```python
from build123d import *

# Parameters (mm, degrees)
SKETCH1_R           = 24.1681
BOSS_EXTRUDE1_DEPTH = 69.7992
SKETCH2_R           = 20.2819
CUT_EXTRUDE1_DEPTH  = 78.718224606
SKETCH3_R           = 4.2164
CUT_EXTRUDE2_DEPTH  = 69.7992
SKETCH4_R           = 4.2164
CUT_EXTRUDE3_DEPTH  = 69.7992


with BuildPart() as part:
    # Sketch1 → Boss-Extrude1 (new body)
    with BuildSketch(Plane(origin=(0, 0, 0), x_dir=(1, 0, 0), z_dir=(0, 1, 0))):
        with Locations(Location((0, 0, 0), (0, 0, 270))):
            Circle(SKETCH1_R)
    extrude(amount=-BOSS_EXTRUDE1_DEPTH)

    # Sketch2 → Cut-Extrude1 (cut, through all)
    with BuildSketch(Plane(origin=(0, 0, 0), x_dir=(1, 0, 0), z_dir=(0, 1, 0))):
        with Locations(Location((0, 0, 0), (0, 0, 270))):
            Circle(SKETCH2_R)
    extrude(amount=-CUT_EXTRUDE1_DEPTH, mode=Mode.SUBTRACT)

    # Sketch3 → Cut-Extrude2 (cut)
    with BuildSketch(Plane.XY):
        with Locations(Location((0, -19.05, 0), (0, 0, 270))):
            Circle(SKETCH3_R)
    extrude(amount=CUT_EXTRUDE2_DEPTH, mode=Mode.SUBTRACT)

    # Sketch4 → Cut-Extrude3 (cut)
    with BuildSketch(Plane(origin=(0, 0, 0), x_dir=(0, 0, -1), z_dir=(1, 0, 0))):
        with Locations(Location((0, -12.7, 0), (0, 0, 180))):
            Circle(SKETCH4_R)
    extrude(amount=CUT_EXTRUDE3_DEPTH, mode=Mode.SUBTRACT)


solid = part.part
```
Can you work these out from the model? Positions are in its coordinate system, mm. A direction names the side the tool comes from. Round coordinates to 2 decimals unless told otherwise and drop trailing zeros. Loops run counter-clockwise (first coordinate to the right, second up) from the corner with the lowest first, then second, coordinate; pieces in that order, holes last. Notation, with made-up numbers: M 62.25,23.5 L 121.25,23.5 A19 cw 121.25,54.5 Z; hole C 16,75.5 d6. An arc over 180 degrees is marked long. Answer as a JSON object with one key per item and string values. Group by question number.
Q1. Please list where these lines run through material, in increasing order: L1, parallel to Y at x = 0, z = 23.1; L2, parallel to Y at x = 20.95, z = 0; L3, parallel to Z at x = -14.5, y = -9.
Q2. Imagine slicing it at D-D, the plane z = 10.5. Please give me the cut outline in (x, y).
Q3. On a 3-axis mill with a long thin cutter (end or side, diameter ignored), from which of +Z, -Z, +X, -X, +Y, -Y can I reach the whole of each face in a straight line? I mean faces 5 (the flat face through (20, -69.799, -5)), 6 (the cylindrical face through (21.972, -10.134, -3.346)). Say none if no direction works.
Q4. Imagine slicing it at B-B, the plane x = 0. Please give me the cut outline in (y, z), then the cut area to 3 significant figures.
Q5. We'd pull the mould along X, two halves only. Please class faces 1 (the cylindrical face through (-23.593, -34.411, -5.239)), 2 (the cylindrical face through (-19.8, -34.4, -4.4)), 3 (the cylindrical face through (3.555, -21.317, 21.973)), 4 (the flat face through (20, 0, -5)): +X half, -X half, draft (parallel to the pull), parting line (faces both ways), or undercut.
Q6. Will these pins go through, and if not, where does the flat tip stop? pin 1 (8 mm diameter, centred on x = 7, y = -32.5, fed in from +Z); pin 2 (3 mm diameter, centred on x = -19, z = 6.5, fed in from -Y); pin 3 (6 mm diameter, centred on x = 7, y = -55.5, fed in from -Z); pin 4 (2 mm diameter, centred on x = -14.5, y = -62, fed in from -Z).
Q7. Imagine slicing it at A-A, the plane z = 0. Please give me the cut outline in (x, y), then the cut area to 3 significant figures.
Q8. Imagine slicing it at C-C, the plane x = -17. Please give me the cut outline in (y, z).
Findings:
{
 "1": {"L1": "y = -69.8 to -23.27, -14.83 to 0", "L2": "y = -69.8 to -16.92, -8.48 to 0", "L3": "z = -19.34 to -14.18, 14.18 to 19.34"},
 "2": {"outline": "M -21.77,-69.8 L -17.35,-69.8 L -17.35,0 L -21.77,0 Z; M 17.35,-69.8 L 21.77,-69.8 L 21.77,0 L 17.35,0 Z"},
 "3": {"face 5": "+Z, -Z, +X, -X, -Y", "face 6": "+X"},
 "4": {"outline": "M -69.8,-24.17 L 0,-24.17 L 0,-20.28 L -69.8,-20.28 Z; M -69.8,20.28 L -23.27,20.28 L -23.27,24.17 L -69.8,24.17 Z; M -14.83,20.28 L 0,20.28 L 0,24.17 L -14.83,24.17 Z", "area": "510 mm2"},
 "5": {"face 1": "parting line", "face 2": "undercut", "face 3": "undercut", "face 4": "draft"},
 "6": {"pin 1": "stops at z = 23.98", "pin 2": "stops at y = -69.8", "pin 3": "stops at z = -23.83", "pin 4": "stops at z = -20.05"},
 "7": {"outline": "M -24.17,-69.8 L -20.28,-69.8 L -20.28,0 L -24.17,0 Z; M 20.28,-69.8 L 24.17,-69.8 L 24.17,-16.92 L 20.28,-16.92 Z; M 20.28,-8.48 L 24.17,-8.48 L 24.17,0 L 20.28,0 Z", "area": "510 mm2"},
 "8": {"outline": "M -69.8,-17.18 L 0,-17.18 L 0,-11.06 L -69.8,-11.06 Z; M -69.8,11.06 L 0,11.06 L 0,17.18 L -69.8,17.18 Z"}
}
